Autodesk Inventor part; units mm, degrees
ref_plane "YZ Plane" through (0, 0, 0) normal (1, 0, 0) x (0, 1, 0)
ref_plane "XZ Plane" through (0, 0, 0) normal (0, 1, 0) x (-1, 0, 0)
ref_plane "XY Plane" through (0, 0, 0) normal (0, 0, 1) x (1, 0, 0)
sketch "Skizze1" plane through (0, 0, 0) normal (0, 1, 0) x (-1, 0, 0)
  line L0 (27.25, -10) -> (27.25, -35.9351) construction
  line L1 (27.25, -35.9351) -> (-27.25, -35.9351) construction
  line L2 (24.25, -10) -> (24.25, 0) construction
  line L3 (46, 4.8366) -> (46, 6.8366)
  line L4 (46, 6.8366) -> (38, 6.8366)
  line L5 (0, 0) -> (0, 30) construction
  line L6 (38, 6.8366) -> (38, 13.8366)
  line L7 (46, 4.8366) -> (27.75, 4.8366)
  line L8 (27.75, 4.8366) -> (27.75, 13.8366)
  line L9 (27.75, 13.8366) -> (23.75, 13.8366)
  line L10 (23.75, 13.8366) -> (23.75, 9.8366)
  line L11 (-46, 4.8366) -> (-46, 6.8366)
  line L12 (-46, 6.8366) -> (-38, 6.8366)
  line L13 (-38, 6.8366) -> (-38, 13.8366)
  line L14 (-46, 4.8366) -> (-27.75, 4.8366)
  line L15 (-27.75, 4.8366) -> (-27.75, 13.8366)
  line L16 (-27.75, 13.8366) -> (-23.75, 13.8366)
  line L17 (-23.75, 13.8366) -> (-23.75, 9.8366)
  arc A0 (38, 13.8366) -> (-38, 13.8366) centre (0, -18.6595) ccw
  line L18 (23.75, 9.8366) -> (-23.75, 9.8366)
  line L19 (0, 9.8366) -> (0, 31.3405)
  point P0 (-27.25, -35.9351)
  dimension "d0" = 2
  dimension "d1" = 7
  dimension "d2" = 8
  dimension "d3" = 46
  dimension "d4" = 0.5
  dimension "d5" = 0.5
  dimension "d7" = 50
  dimension "d8" = 9
  dimension "d9" = 4
  dimension "d11" = 26.5038
revolve "Umdrehung1" add sketch "Skizze1" angle 360 about axis through (0, 0, 9.8366) along (0, 0, 1) contours L7 L8 L9 L10 L18 L19 A0 L6 L4 L3
Here's how the part is built. I have some questions about the finished solid (model axes, mm). A direction names the side the tool comes from. Give positions to 0.01 mm unless a question says otherwise; leave off trailing zeros. Write each loop counter-clockwise with the first axis right and the second up, starting at its lowest first coordinate (ties: lowest second). Pieces come first, ordered by that corner, then holes. Notation, with made-up numbers: (-0.75, 54.5) -> (32.25, 54.5) arc R26 ccw to (32.25, 85.5) -> close; hole circle Ø5 at (42.25, 83.5). An arc over 180 degrees is marked (long way). Use one line per item in the form item = value.
1) Suppose I cut it at B-B (y = 0). Please give me the cut outline in (x, z).
Verdict:
outline = (-46, 4.84) -> (-27.75, 4.84) -> (-27.75, 13.84) -> (-23.75, 13.84) -> (-23.75, 9.84) -> (23.75, 9.84) -> (23.75, 13.84) -> (27.75, 13.84) -> (27.75, 4.84) -> (46, 4.84) -> (46, 6.84) -> (38, 6.84) -> (38, 13.84) arc R50 ccw to (-38, 13.84) -> (-38, 6.84) -> (-46, 6.84) -> close
2) Suppose I cut it at D-D (x = 34). Please give me the cut outline in (y, z), and give its area (3 significant figures).
Verdict:
outline = (-30.98, 4.84) -> (30.98, 4.84) -> (30.98, 6.84) -> (16.97, 6.84) -> (16.97, 13.84) arc R36.66 ccw to (-16.97, 13.84) -> (-16.97, 6.84) -> (-30.98, 6.84) -> close
area = 457 mm2
3) I'm going to push flat-ended pins straight in: pin 1 (3 mm diameter, centred on x = -16.5, y = -15, fed in from +Z); pin 2 (8 mm diameter, centred on y = -7, z = 14, fed in from +X); pin 3 (10 mm diameter, centred on y = -8.5, z = 23.5, fed in from -X). Where does each tip first touch, or does it pass through?
Verdict:
pin_1 = 26.81
pin_2 = 37.88
pin_3 = -32.49
4) If I drill on L1, parallel to Y at x = 0, z = 10.5; L2, parallel to X at y = 0, z = 9, over which ranges is the centre line in solid material (lowest first)? Write a range as [from, to].
Verdict:
L1 = [-38, -27.75], [-23.75, 23.75], [27.75, 38]
L2 = [-38, -27.75], [27.75, 38]
5) We'd pull the mould along X, two halves only. Please class faces 4 (the face through (0, 0, 9.837)), 5 (the face through (-7, -38, 6.837)), 6 (the face through (5.99, -45.61, 5.85)): +X half, -X half, draft (parallel to the pull), parting line (faces both ways), or undercut.
Verdict:
face_4 = undercut
face_5 = draft
face_6 = parting line
6) On a 3-axis mill with a long thin cutter (end or side, diameter ignored), from which of +Z, -Z, +X, -X, +Y, -Y can I reach the whole of each face in a straight line? I mean faces 1 (the face through (-20, 20, 4.837)), 2 (the face through (-20.4, -12.5, 13.837)), 3 (the face through (-17.535, 33.713, 10.386)). Say none if no direction works.
Verdict:
face_1 = -Z, +X, -X, +Y, -Y
face_2 = -Z
face_3 = +Z
7) Suppose I cut it at A-A (z = 12.75). Please give me the cut outline in (x, y).
Verdict:
outline = circle Ø76 at (0, 0); circle Ø47.5 at (0, 0); hole circle Ø55.5 at (0, 0)
